```python
from build123d import *

# Parameters (mm, degrees)
SKETCH3_R           = 11
BOSS_EXTRUDE1_DEPTH = 5
SKETCH4_R           = 10.1
BOSS_EXTRUDE2_DEPTH = 11
SKETCH5_R           = 2.7
CUT_EXTRUDE1_DEPTH  = 17


with BuildPart() as part:
    # Sketch3 → Boss-Extrude1 (new body)
    with BuildSketch(Plane.XY):
        Circle(SKETCH3_R)
    extrude(amount=BOSS_EXTRUDE1_DEPTH)

    # Sketch4 → Boss-Extrude2 (add)
    with BuildSketch(Plane(origin=(0, 0, 0), x_dir=(-1, 0, 0), z_dir=(0, 0, -1))):
        Circle(SKETCH4_R)
    extrude(amount=BOSS_EXTRUDE2_DEPTH)

    # Sketch5 → Cut-Extrude1 (cut, through all)
    with BuildSketch(Plane.XY.offset(5)):
        Circle(SKETCH5_R)
    extrude(amount=-CUT_EXTRUDE1_DEPTH, mode=Mode.SUBTRACT)


solid = part.part
```
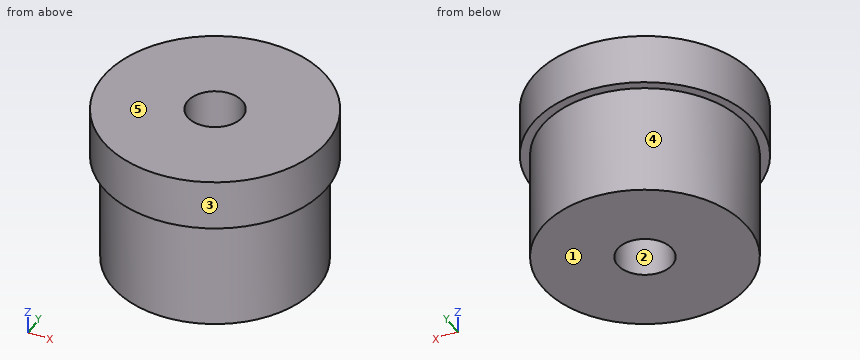
CAD build for the part. Positions are in the model's coordinates, mm. Face numbers are marked on the shaded views. A direction names the side the tool comes from. Coordinates: 2 decimals unless noted, no trailing zeros. Order: outer loops, then holes, each group sorted by start corner. A loop starts at its lowest first (then second) coordinate and runs counter-clockwise, first axis right, second up. Notation, with made-up numbers: (-12, 87) - (-6, 87) arc R24 cw to (-6, 102) - close; hole circle Ø10 at (86.25, 87.25). An arc over 180 degrees is marked (long way). Answer in a Markdown table with one row per item.
1. Drill centre lines: L1, parallel to Y at x = 0, z = -1.25; L2, parallel to Y at x = 0, z = 1.75; L3, parallel to X at y = -1.75, z = -5.5. Where is each one in solid material? Low to high. Write a range as from..to.
Answer:
| item | result |
|---|---|
| L1 | -10.1..-2.7, 2.7..10.1 |
| L2 | -11..-2.7, 2.7..11 |
| L3 | -9.95..-2.06, 2.06..9.95 |
2. Pull direction Y, two halves, no side cores. Call the marked faces 1, 2 and 3: +Y half, -Y half, draft (parallel to the pull), parting line (faces both ways), or undercut.
Answer:
| item | result |
|---|---|
| face 1 | draft |
| face 2 | undercut |
| face 3 | parting line |
3. Slice it at D-D, the plane y = 4. List the corners of the cut face in (x, z), then the cut area to 3 significant figures.
Answer:
| item | result |
|---|---|
| outline | (-10.25, 0) - (-9.27, 0) - (-9.27, -11) - (9.27, -11) - (9.27, 0) - (10.25, 0) - (10.25, 5) - (-10.25, 5) - close |
| area | 307 mm² |
4. Flat gauge pins, fed straight in: P1, Ø6, axis at x = 0, y = 0, coming from the +Z side; P2, Ø1, axis at y = 5.5, z = 0.5, coming from the +X side; P3, Ø1.5, axis at y = -5, z = -9.5, coming from the -X side; P4, Ø1.5, axis at y = 1, z = 1.5, coming from the -X side. Where does each tip first touch, or does it go through?
Answer:
| item | result |
|---|---|
| P1 | z = 5 |
| P2 | x = 9.8 |
| P3 | x = -9.16 |
| P4 | x = -11 |
5. Slice it at A-A, the plane y = 0. List the corners of the cut face in (x, z).
Answer:
| item | result |
|---|---|
| outline | (-11, 0) - (-10.1, 0) - (-10.1, -11) - (-2.7, -11) - (-2.7, 5) - (-11, 5) - close; (2.7, -11) - (10.1, -11) - (10.1, 0) - (11, 0) - (11, 5) - (2.7, 5) - close |
6. Slice it at C-C, the plane z = -1.5. List the corners of the cut face in (x, y).
Answer:
| item | result |
|---|---|
| outline | circle Ø20.2 at (0, 0); hole circle Ø5.4 at (0, 0) |
7. 3-axis set-ups, long thin cutter, end or side, ignore diameter. For the marked faces 4 and 5: which of +Z, -Z, +X, -X, +Y, -Y reach the whole face in a straight line?
Answer:
| item | result |
|---|---|
| face 4 | -Z |
| face 5 | +Z, +X, -X, +Y, -Y |
